Could you check a few things on this model? Use its own coordinates, in mm. Face numbers are marked on the shaded views. Coordinates: 2 decimals unless noted, no trailing zeros. Write each loop counter-clockwise with the first axis right and the second up, starting at its lowest first coordinate (ties: lowest second). Pieces come first, ordered by that corner, then holes.
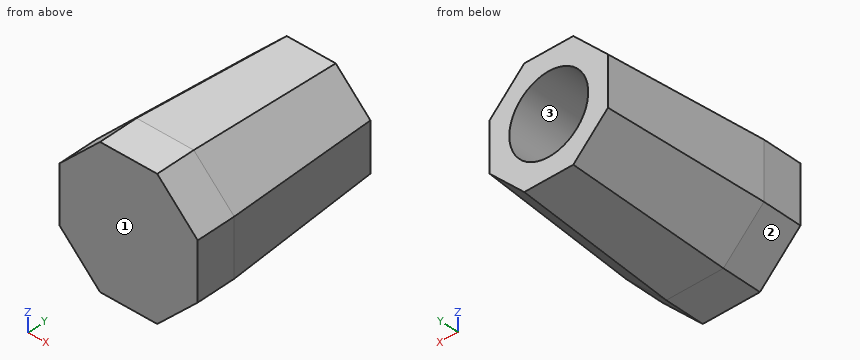
Autodesk Inventor part; units mm, degrees
ref_plane "YZ Plane" through (0, 0, 0) normal (1, 0, 0) x (0, 1, 0)
ref_plane "XZ Plane" through (0, 0, 0) normal (0, 1, 0) x (-1, 0, 0)
ref_plane "XY Plane" through (0, 0, 0) normal (0, 0, 1) x (1, 0, 0)
sketch "Sketch1" plane through (0, 0, 0) normal (0, 1, 0) x (-1, 0, 0)
  line L0 (7.8908, 19.05) -> (19.05, 7.8908)
  line L1 (19.05, 7.8908) -> (19.05, -7.8908)
  line L2 (19.05, -7.8908) -> (7.8908, -19.05)
  line L3 (7.8908, -19.05) -> (-7.8908, -19.05)
  line L4 (-7.8908, -19.05) -> (-19.05, -7.8908)
  line L5 (-19.05, -7.8908) -> (-19.05, 7.8908)
  line L6 (-19.05, 7.8908) -> (-7.8908, 19.05)
  line L7 (-7.8908, 19.05) -> (7.8908, 19.05)
  point P0 (0, 0)
  point P1 (0, 0)
  dimension "d5" = 19.05
extrude "Extrusion1" add sketch "Sketch1" against normal blind 50.8
sketch "Sketch4" plane through (0, -50.8, 0) normal (0, -1, 0) x (1, 0, 0)
  line L0 (9.2059, 22.225) -> (22.225, 9.2059)
  line L1 (22.225, 9.2059) -> (22.225, -9.2059)
  line L2 (22.225, -9.2059) -> (9.2059, -22.225)
  line L3 (9.2059, -22.225) -> (-9.2059, -22.225)
  line L4 (-9.2059, -22.225) -> (-22.225, -9.2059)
  line L5 (-22.225, -9.2059) -> (-22.225, 9.2059)
  line L6 (-22.225, 9.2059) -> (-9.2059, 22.225)
  line L7 (-9.2059, 22.225) -> (9.2059, 22.225)
  line L8 (7.8908, 19.05) -> (-7.8908, 19.05)
  point P0 (0, 0)
  point P1 (0, 0)
  dimension "d17" = 3.175
loft "Loft1" add profiles "Sketch4" section 2 edges at (-13.4704, 0, 13.4704) (0, 0, 19.05) (13.4704, 0, 13.4704) (19.05, 0, 0) (13.4704, 0, -13.4704) (0, 0, -19.05) (-13.4704, 0, -13.4704) (-19.05, 0, 0)
sketch "Sketch5" plane through (0, 0, 0) normal (0, 1, 0) x (1, 0, 0)
  circle A0 centre (0, 0) radius 12.7
  dimension "d11" = 25.4
extrude "Extrusion2" cut sketch "Sketch5" against normal blind 50.8
ref_plane "Work Plane1" through (0, -50.8, 22.225) normal (1, 0, 0) x (0, 1, 0)
sketch "Sketch6" plane through (0, -50.8, 22.225) normal (1, 0, 0) x (0, 1, 0)
  point P0 (50.8, -22.225)
sketch "Sketch7" plane through (0, -50.8, 22.225) normal (1, 0, 0) x (0, 1, 0)
  point P0 (50.8, -22.225)
sketch "Sketch8" plane through (0, -50.8, 0) normal (0, -1, 0) x (1, 0, 0)
  circle A0 centre (0, 0) radius 12.7
  line L0 (9.2059, 22.225) -> (22.225, 9.2059)
  line L1 (-9.2059, 22.225) -> (9.2059, 22.225)
  line L2 (-22.225, 9.2059) -> (-9.2059, 22.225)
  line L3 (-22.225, -9.2059) -> (-22.225, 9.2059)
  line L4 (-9.2059, -22.225) -> (-22.225, -9.2059)
  line L5 (9.2059, -22.225) -> (-9.2059, -22.225)
  line L6 (22.225, -9.2059) -> (9.2059, -22.225)
  line L7 (22.225, 9.2059) -> (22.225, -9.2059)
extrude "Extrusion3" add sketch "Sketch8" along normal blind 12.7 contours A0 | L0 L7 L6 L5 L4 L3 L2 L1
sketch "Sketch9" plane through (0, -50.8, 22.225) normal (1, 0, 0) x (0, 1, 0)
  line L0 (-12.7, -31.4309) -> (-12.7, -44.45) construction
  line L1 (-12.7, -13.0191) -> (-12.7, -31.4309) construction
  line L2 (-12.7, 0) -> (-12.7, -13.0191) construction
  line L3 (0, -44.45) -> (-12.7, -44.45) construction
  line L4 (0, -44.45) -> (50.8, -41.275) construction
  line L5 (0, 0) -> (-12.7, 0) construction
  line L6 (0, 0) -> (50.8, -3.175) construction
  line L7 (0, -13.0191) -> (0, 0) construction
  line L8 (0, -34.925) -> (0, -9.525) construction
  line L9 (0, -44.45) -> (0, -31.4309) construction
  line L10 (50.8, -30.1158) -> (50.8, -41.275) construction
  line L11 (50.8, -9.525) -> (50.8, -34.925) construction
  line L12 (50.8, -3.175) -> (50.8, -14.3342) construction
  line L13 (-6.35, 0) -> (-6.35, -44.45) construction
  line L14 (-12.7, -22.225) -> (0, -22.225) construction
  arc A0 (-37.0757, -22.225) -> (-31.6983, -79.4354) centre (269.9482, -22.225) ccw
  line L15 (-37.0757, -22.225) -> (-6.35, -22.225)
  arc A1 (-6.35, -44.45) -> (-24.1759, -60.6977) centre (-5.386, -63.4102) ccw
  point P0 (50.8, -22.225)
properties part number "V1.0"
1. For pin 1 (12.5 mm diameter, centred on x = 3.5, z = -2.5, fed in from +Y); pin 2 (2 mm diameter, centred on y = -33, z = 13, fed in from +X); pin 3 (10 mm diameter, centred on x = 13, y = -16, fed in from +Z), each with a flat end and sliding along its axis, tell me the tip position at first contact or that it passes through.
Verdict:
pin 1: stops at y = -50.8
pin 2: stops at x = 17.86
pin 3: stops at z = 20.17
2. If we mould it in two halves opening along X, with no side actions, what happens to the marked faces 1, 2 and 3? For each: pulls with the +X half, pulls with the -X half, needs draft (parallel to the pull), parting line crosses it, or undercut.
Verdict:
face 1: needs draft
face 2: pulls with the -X half
face 3: undercut
3. I want a section at A-A on y = -56. Please give me the cut outline in (x, z) (3 decimals).
Verdict:
outline: (-22.225, -9.206) - (-9.206, -22.225) - (9.206, -22.225) - (22.225, -9.206) - (22.225, 9.206) - (9.206, 22.225) - (-9.206, 22.225) - (-22.225, 9.206) - close
4. Please list where these lines run through material, in increasing order: line 1 along Y through (x, z) = (-6.5, 8); line 2 along Z through (x, y) = (0, -15.5); line 3 along Z through (x, y) = (0, -24).
Verdict:
line 1: y = -63.5 to -50.8
line 2: z = -20.02 to -12.7, 12.7 to 20.02
line 3: z = -20.55 to -12.7, 12.7 to 20.55
